Source: CAD feature listing. Evaluate the final solid. Frame: model axes, mm. Face numbers are marked on the shaded views. A direction names the side the tool comes from. Give positions to 0.01 mm unless a question says otherwise; leave off trailing zeros. Write each loop counter-clockwise with the first axis right and the second up, starting at its lowest first coordinate (ties: lowest second). Pieces come first, ordered by that corner, then holes. Notation, with made-up numbers: (-5, -9) -> (12, -9) arc R33 cw to (12, 22) -> close; hole circle Ø8 at (-6, -32). An arc over 180 degrees is marked (long way). Use one line per item in the form item = value. Start each with the question number.
(1) Draft query along Y for the marked faces 4, 5, 6 and 7. Return one class per face: pulls with the +Y half, pulls with the -Y half, needs draft (parallel to the pull), parting line crosses it, or undercut.
(2) Material intervals for line 1 along Y through (x, z) = (29, 0); line 2 along Y through (x, z) = (33, 0); line 3 along X through (y, z) = (12.5, 3), sorted ascending. Write a range as from..to.
(3) First-contact query: P1, Ø15, axis at y = -0.5, z = 8.5, coming from the +X side; P2, Ø5, axis at x = -42.5, z = 2.5, coming from the -Y side; P3, Ø1, axis at x = -13.5, z = 1.5, coming from the -Y side; P4, Ø1.5, axis at y = -4.5, z = 3, coming from the +X side. Flat tips, straight axial feed; report the tip coordinate or a pass-through.
(4) Set-up query: the marked faces 1, 2 and 3. Return all of +Z, -Z, +X, -X, +Y, -Y with unobstructed straight access to the full face (end or side cutting, diameter ignored); none if empty.
(5) Cut plane B-B, the plane x = -55.5. Output: boundary loops of the cut face in (y, z).
(6) Cut plane A-A, the plane x = -13. Output: boundary loops of the cut face in (y, z).
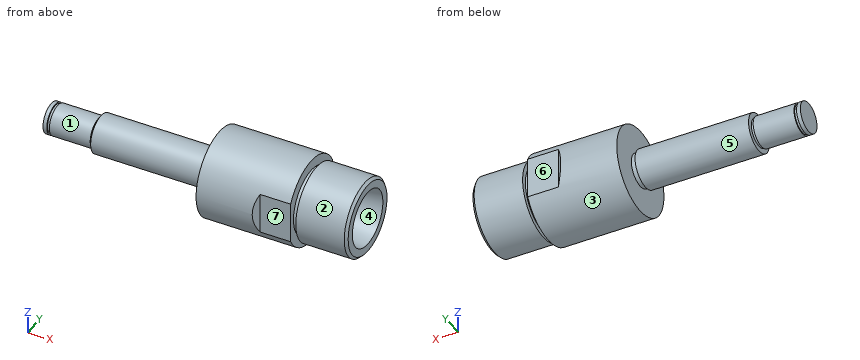
from build123d import *

# Parameters (mm, degrees)
SKETCH_4_OUTSIDE_W  = 62.6
SKETCH_4_OUTSIDE_H  = 62.6
CUT_EXTRUDE_2_DEPTH = 14
CHAMFER_1_SIZE      = 2
CHAMFER_2_SIZE      = 1


with BuildPart() as part:
    # 草图1 → 旋转1 (revolve)
    with BuildSketch(Plane.XY, mode=Mode.PRIVATE) as revolve_1_sk:
        Polygon((0, 6.5), (0, 17), (36, 17), (36, 13), (38, 13), (38, 15), (58, 15), (58, 11), (42, 8.680110408), (42, 9.5), (37, 9.5), (37, 9), (31, 9), (31, 9.5), (26, 9.5), (26, 7), (10, 7), (5.793975667, 0), (-66, 0), (-66, 6), (-64.5, 6), (-64.5, 5.5), (-63.5, 5.5), (-63.5, 6), (-47.5, 6), (-47.5, 5.5), (-46.5, 5.5), (-46.5, 7.5), (-2, 7.5), (-2, 6.5), align=None)
    revolve(revolve_1_sk.sketch.rotate(Axis((-14.714771185, 0, 0), (1, 0, 0)), 90), axis=Axis((-14.714771185, 0, 0), (1, 0, 0)))

    # 草图4 outside → 切除-拉伸2 (cut)
    with BuildSketch(Plane(origin=(36, 0, 0), x_dir=(0, 0, -1), z_dir=(1, 0, 0))):
        Rectangle(SKETCH_4_OUTSIDE_W, SKETCH_4_OUTSIDE_H)
        with BuildLine():
            Line((-8, -15), (8, -15))
            ThreePointArc((8, -15), (17, 0), (8, 15))
            Line((8, 15), (-8, 15))
            ThreePointArc((-8, 15), (-17, 0), (-8, -15))
        make_face(mode=Mode.SUBTRACT)
    extrude(amount=-CUT_EXTRUDE_2_DEPTH, mode=Mode.SUBTRACT)

    # 倒角1
    chamfer_1_edges = [part.edges().sort_by_distance(p)[0] for p in [
        (22, -15, 0),
        (22, 15, 0),
    ]]
    chamfer(chamfer_1_edges, length=CHAMFER_1_SIZE - 0.0001)  # a hair under: the kernel refuses the full size

    # 倒角2
    chamfer_2_edges = [part.edges().sort_by_distance(p)[0] for p in [
        (58, 0, -15),
    ]]
    chamfer(chamfer_2_edges, length=CHAMFER_2_SIZE)


solid = part.part
Geometry says:
q1.face_4 = undercut
q1.face_5 = parting line crosses it
q1.face_6 = pulls with the +Y half
q1.face_7 = pulls with the -Y half
q2.line_1 = -15..-9.5, 9.5..15
q2.line_2 = -15..-9, 9..15
q2.line_3 = 0..58
q3.P1 = 58
q3.P2 = -7.5
q3.P3 = -7.43
q3.P4 = 9.49
q4.face_1 = -X
q4.face_2 = +X
q4.face_3 = +X, -X
q5.outline = circle Ø12 at (0, 0)
q6.outline = circle Ø15 at (0, 0)
